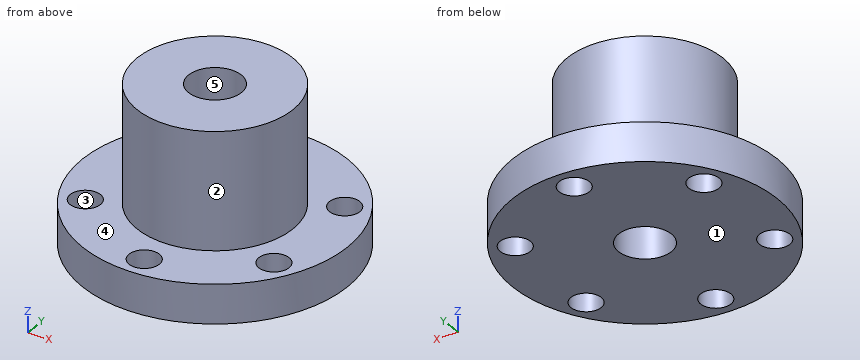
```python
from build123d import *

# Parameters (mm, degrees)
TALADRO_ROSCADO_M81_D     = 6.8
TALADRO_ROSCADO_M81_DEPTH = 22.25
TALADRO_ROSCADO_M81_TIP   = 2.042926105
MATRIZC1_COUNT            = 6


with BuildPart() as part:
    # Croquis1 → Revolución1 (revolve)
    with BuildSketch(Plane(origin=(0, 0, 0), x_dir=(1, 0, 0), z_dir=(0, 1, 0))):
        Polygon((0, 0), (17, 0), (17, -5), (10, -5), (10, -20), (0, -20), align=None)
    revolve(axis=Axis((0, 0, 0), (0, 0, -1)))

    # Taladro roscado M81
    with Locations(Plane.XY.offset(20)):
        with Locations((0, 0)):
            Hole(TALADRO_ROSCADO_M81_D / 2, depth=TALADRO_ROSCADO_M81_DEPTH)
            with Locations((0, 0, -(TALADRO_ROSCADO_M81_DEPTH + TALADRO_ROSCADO_M81_TIP / 2))):  # 118° drill point
                Cone(0, TALADRO_ROSCADO_M81_D / 2, TALADRO_ROSCADO_M81_TIP, mode=Mode.SUBTRACT)

    # Croquis4 → Taladro de margen para M3.51 (revolve, cut)
    with BuildSketch(Plane(origin=(0, 14, 0), x_dir=(0, 1, 0), z_dir=(1, 0, 0))):
        Polygon((0, 0), (0, 501.171678207), (1.95, 500), (1.95, 0), align=None)
    taladro_de_margen_para_m3_51 = revolve(axis=Axis((0, 14, -6.35), (0, 0, 1)), mode=Mode.SUBTRACT)

    # MatrizC1: Taladro de margen para M3.51 ×6 about axis
    matrizc1_axis = Axis((0, 0, 0), (0, 0, 1))
    for i in range(1, MATRIZC1_COUNT):
        add(taladro_de_margen_para_m3_51.rotate(matrizc1_axis, i * 360 / MATRIZC1_COUNT), mode=Mode.SUBTRACT)


solid = part.part
```
For this review, take the finished solid that the model builds, in its own axes (mm). Face numbers are marked on the shaded views. A direction names the side the tool comes from. Coordinates: 2 decimals unless noted, no trailing zeros. Write each loop counter-clockwise with the first axis right and the second up, starting at its lowest first coordinate (ties: lowest second). Pieces come first, ordered by that corner, then holes. Notation, with made-up numbers: (34.5, 30) -> (40.5, 30) arc R27 ccw to (40.5, 59) -> close; hole circle Ø5 at (83.5, 52.5). An arc over 180 degrees is marked (long way). Put each result on its own line as item: value.
Q1. Clearance check with flat-ended pins moving along their axes: pin 1 Ø12 at (x, z) = (8, 16.5) entering from +Y; pin 2 Ø2 at (y, z) = (-11, 5.5) entering from -X; pin 3 Ø1 at (y, z) = (-7, 8.5) entering from +X. State where each tip first meets the part, or that it passes through.
From the geometry:
pin 1: stops at y = 9.8
pin 2: stops at x = -13.65
pin 3: stops at x = 7.6
Q2. The part is to be moulded in two halves that separate along X. For the marked faces 1, 2 and 3, say which applies: +X half, -X half, draft (parallel to the pull), parting line (faces both ways), or undercut.
From the geometry:
face 1: draft
face 2: parting line
face 3: undercut
Q3. Wall thickness on L1, parallel to X at y = -1, z = 2.5; L2, parallel to Z at x = -15, y = 3; L3, parallel to X at y = -3, z = 14.5: over which ranges is each line inside the solid? List them lowest first.
From the geometry:
L1: x = -16.97 to -3.25, 3.25 to 16.97
L2: z = 0 to 5
L3: x = -9.54 to -1.6, 1.6 to 9.54
Q4. Take a section at A-A, the plane x = 0. State the section outline as (y, z) points.
From the geometry:
outline: (-17, 0) -> (-15.95, 0) -> (-15.95, 5) -> (-17, 5) -> close; (-12.05, 0) -> (-3.4, 0) -> (-3.4, 20) -> (-10, 20) -> (-10, 5) -> (-12.05, 5) -> close; (3.4, 0) -> (12.05, 0) -> (12.05, 5) -> (10, 5) -> (10, 20) -> (3.4, 20) -> close; (15.95, 0) -> (17, 0) -> (17, 5) -> (15.95, 5) -> close
Q5. Take a section at D-D, the plane y = 7. State the section outline as (x, z) points, then the cut area to 3 significant figures.
From the geometry:
outline: (-15.49, 0) -> (-14.07, 0) -> (-14.07, 5) -> (-15.49, 5) -> close; (-10.17, 0) -> (10.17, 0) -> (10.17, 5) -> (7.14, 5) -> (7.14, 20) -> (-7.14, 20) -> (-7.14, 5) -> (-10.17, 5) -> close; (14.07, 0) -> (15.49, 0) -> (15.49, 5) -> (14.07, 5) -> close
area: 330 mm2
Q6. Take a section at C-C, the plane z = 7.25. State the section outline as (x, y) points, then the cut area to 3 significant figures.
From the geometry:
outline: circle Ø20 at (0, 0); hole circle Ø6.8 at (0, 0)
area: 278 mm2
Q7. Take a section at B-B, the plane y = 0. State the section outline as (x, z) points.
From the geometry:
outline: (-17, 0) -> (-3.4, 0) -> (-3.4, 20) -> (-10, 20) -> (-10, 5) -> (-17, 5) -> close; (3.4, 0) -> (17, 0) -> (17, 5) -> (10, 5) -> (10, 20) -> (3.4, 20) -> close
Q8. Tool access review of the marked faces 4 and 5: name each direction out of +Z, -Z, +X, -X, +Y, -Y from which nothing blocks a thin tool from reaching the whole face with its end or side.
From the geometry:
face 4: +Z
face 5: +Z, -Z
